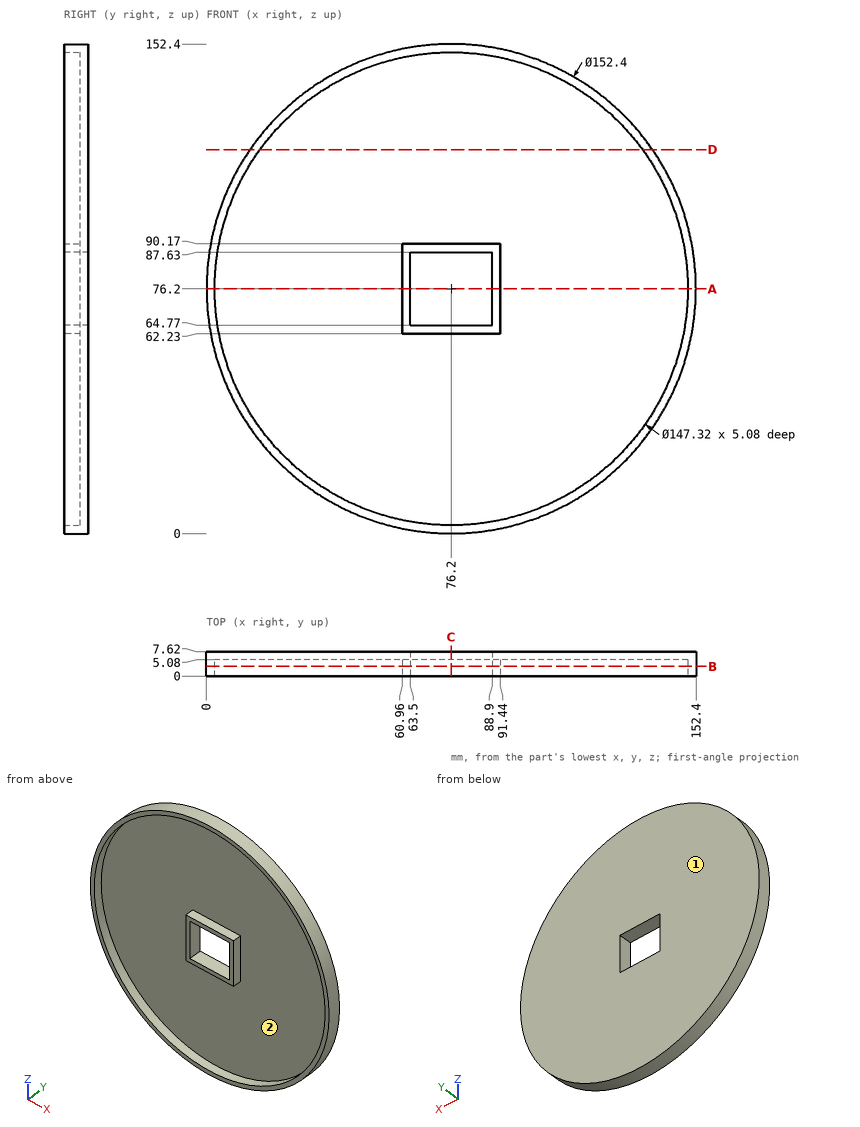
Answer from the drawing. Dimensions are ordinates in mm from the lowest x, y and z of the part. Coordinates: 2 decimals unless noted, no trailing zeros. Loops run counter-clockwise (first coordinate to the right, second up) from the corner with the lowest first, then second, coordinate; pieces in that order, holes last. Notation, with made-up numbers: (47, -29) - (71, -29) arc R22 cw to (71, 10) - close; hole circle Ø11 at (34, 5). An arc over 180 degrees is marked (long way). Answer in a Markdown table with one row per item.
1. Straight lines are drawn through the part: line 1 (Z direction, x = 76.2, y = 1.65); line 2 (Z direction, x = 64.5, y = 5); line 3 (Y direction, x = 127, z = 65). For each, find the intervals that lie inside material, in ascending order.
Conclusion:
| item | result |
|---|---|
| line 1 | z = 0 to 2.54, 62.23 to 64.77, 87.63 to 90.17, 149.86 to 152.4 |
| line 2 | z = 0.9 to 3.48, 62.23 to 64.77, 87.63 to 90.17, 148.92 to 151.5 |
| line 3 | y = 5.08 to 7.62 |
2. Find section D-D, the plane z = 119.5. Write down the section's boundary in (x, y), then the cut area to 3 significant figures.
Conclusion:
| item | result |
|---|---|
| outline | (13.5, 0) - (16.61, 0) - (16.61, 5.08) - (135.79, 5.08) - (135.79, 0) - (138.9, 0) - (138.9, 7.62) - (13.5, 7.62) - close |
| area | 350 mm² |
3. Determine the mould class of the marked faces 1 and 2 for opening direction Z: +Z half, -Z half, draft (parallel to the pull), parting line (faces both ways), or undercut.
Conclusion:
| item | result |
|---|---|
| face 1 | draft |
| face 2 | undercut |
4. Given pin 1 (4 mm diameter, centred on y = 4.5, z = 75, fed in from +X); pin 2 (3 mm diameter, centred on x = 78.5, y = 4.5, fed in from -Z); pin 3 (12 mm diameter, centred on x = 88, z = 47.5, fed in from -Y); pin 4 (2.5 mm diameter, centred on y = 4.5, z = 72, fed in from -X), each flat-ended and moving along its own axis, determine where each tip first touches the part or whether it passes through.
Conclusion:
| item | result |
|---|---|
| pin 1 | stops at x = 152.4 |
| pin 2 | stops at z = 0 |
| pin 3 | stops at y = 5.08 |
| pin 4 | stops at x = 0.06 |
5. Find section A-A, the plane z = 76.2. Write down the section's boundary in (x, y).
Conclusion:
| item | result |
|---|---|
| outline | (0, 0) - (2.54, 0) - (2.54, 5.08) - (60.96, 5.08) - (60.96, 0) - (63.5, 0) - (63.5, 7.62) - (0, 7.62) - close; (88.9, 0) - (91.44, 0) - (91.44, 5.08) - (149.86, 5.08) - (149.86, 0) - (152.4, 0) - (152.4, 7.62) - (88.9, 7.62) - close |
6. Find section C-C, the plane x = 76.2. Write down the section's boundary in (y, z).
Conclusion:
| item | result |
|---|---|
| outline | (0, 0) - (7.62, 0) - (7.62, 64.77) - (0, 64.77) - (0, 62.23) - (5.08, 62.23) - (5.08, 2.54) - (0, 2.54) - close; (0, 87.63) - (7.62, 87.63) - (7.62, 152.4) - (0, 152.4) - (0, 149.86) - (5.08, 149.86) - (5.08, 90.17) - (0, 90.17) - close |
7. Find section B-B, the plane y = 3. Write down the section's boundary in (x, z), then the cut area to 3 significant figures.
Conclusion:
| item | result |
|---|---|
| outline | circle Ø152.4 at (76.2, 76.2); (60.96, 62.23) - (91.44, 62.23) - (91.44, 90.17) - (60.96, 90.17) - close; hole circle Ø147.32 at (76.2, 76.2); hole (63.5, 64.77) - (88.9, 64.77) - (88.9, 87.63) - (63.5, 87.63) - close |
| area | 1,470 mm² |
